Model file for the job. Use its own axes, mm. Round coordinates to 2 decimals unless told otherwise and drop trailing zeros. Write each loop counter-clockwise with the first axis right and the second up, starting at its lowest first coordinate (ties: lowest second). Pieces come first, ordered by that corner, then holes. Notation, with made-up numbers: (-29, 36) - (15, 36) arc R24 ccw to (15, 49) - close; hole circle Ø7 at (58, 62.5). An arc over 180 degrees is marked (long way). Answer as a JSON object with one key per item and string values. Group by question number.
from build123d import *

# Parameters (mm, degrees)
SKETCH1_R           = 0.4445
BOSS_EXTRUDE1_DEPTH = 1.5875


with BuildPart() as part:
    # Sketch1 → Boss-Extrude1 (new body)
    with BuildSketch(Plane.XY):
        Polygon((12.192, 0), (-12.192, 0), (-12.192, 21.082), (-4.5974, 27.6098), (4.5974, 27.6098), (12.192, 21.082), align=None)
        with Locations((-10.9982, 1.628621929)):
            Circle(SKETCH1_R, mode=Mode.SUBTRACT)
        with Locations((-10.9982, 3.660621929)):
            Circle(SKETCH1_R, mode=Mode.SUBTRACT)
        with Locations((-10.9982, 5.692621929)):
            Circle(SKETCH1_R, mode=Mode.SUBTRACT)
        with Locations((-10.9982, 7.724621929)):
            Circle(SKETCH1_R, mode=Mode.SUBTRACT)
        with Locations((-10.9982, 9.756621929)):
            Circle(SKETCH1_R, mode=Mode.SUBTRACT)
        with Locations((-10.9982, 11.788621929)):
            Circle(SKETCH1_R, mode=Mode.SUBTRACT)
        with Locations((-10.9982, 13.820621929)):
            Circle(SKETCH1_R, mode=Mode.SUBTRACT)
        with Locations((-10.9982, 15.852621929)):
            Circle(SKETCH1_R, mode=Mode.SUBTRACT)
        with Locations((-10.9982, 17.884621929)):
            Circle(SKETCH1_R, mode=Mode.SUBTRACT)
        with Locations((-10.9982, 19.916621929)):
            Circle(SKETCH1_R, mode=Mode.SUBTRACT)
        with Locations((10.9982, 19.916621929)):
            Circle(SKETCH1_R, mode=Mode.SUBTRACT)
        with Locations((10.9982, 17.884621929)):
            Circle(SKETCH1_R, mode=Mode.SUBTRACT)
        with Locations((10.9982, 15.852621929)):
            Circle(SKETCH1_R, mode=Mode.SUBTRACT)
        with Locations((10.9982, 13.820621929)):
            Circle(SKETCH1_R, mode=Mode.SUBTRACT)
        with Locations((10.9982, 11.788621929)):
            Circle(SKETCH1_R, mode=Mode.SUBTRACT)
        with Locations((10.9982, 9.756621929)):
            Circle(SKETCH1_R, mode=Mode.SUBTRACT)
        with Locations((10.9982, 7.724621929)):
            Circle(SKETCH1_R, mode=Mode.SUBTRACT)
        with Locations((10.9982, 5.692621929)):
            Circle(SKETCH1_R, mode=Mode.SUBTRACT)
        with Locations((10.9982, 3.660621929)):
            Circle(SKETCH1_R, mode=Mode.SUBTRACT)
        with Locations((10.9982, 1.628621929)):
            Circle(SKETCH1_R, mode=Mode.SUBTRACT)
    extrude(amount=BOSS_EXTRUDE1_DEPTH)


solid = part.part
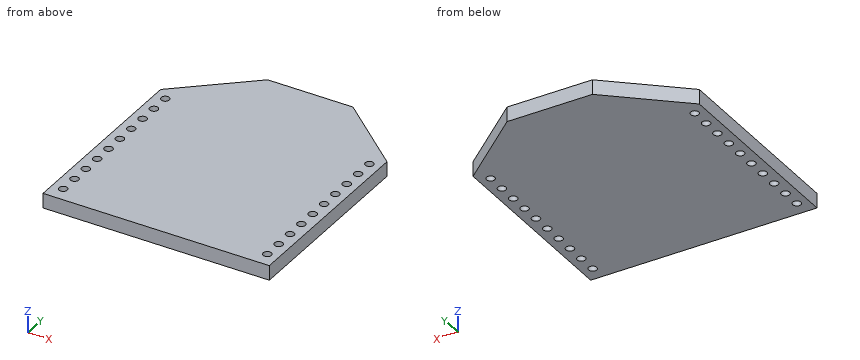
(1) Slice it at A-A (z = 0.4). Count the separate pieces of the cut face and the enclosed holes in it, then the cut area to 3 significant figures.
(2) Drill centre lines: line 1 (X direction, y = 2, z = 1.5); line 2 (X direction, y = 11.5, z = 0.3); line 3 (Y direction, x = 10.5, z = 1.35). Where is each one in solid material? Low to high. Write a range as from..to.
(3) Slice it at C-C (y = 22). Write the cut outline in (x, z), then the cut area to 3 significant figures.
(4) Slice it at B-B (x = 8). Write the cut outline in (y, z), then the cut area to 3 significant figures.
Answer:
{
 "1": {"separate pieces": "1", "enclosed holes": "20", "area": "611 mm²"},
 "2": {"line 1": "-12.19..-11.24, -10.75..10.75, 11.24..12.19", "line 2": "-12.19..-11.34, -10.66..10.66, 11.34..12.19", "line 3": "0..22.54"},
 "3": {"outline": "(-11.12, 0) - (11.12, 0) - (11.12, 1.59) - (-11.12, 1.59) - close", "area": "35.3 mm²"},
 "4": {"outline": "(0, 0) - (24.69, 0) - (24.69, 1.59) - (0, 1.59) - close", "area": "39.2 mm²"}
}
